from build123d import *

# Parameters (mm, degrees)
F1_DEPTH = 38.1
F3_DEPTH = 6.35


# Not quite as in the source:
# - the program builds the solid bodies; features that only make, move or delete a surface that nothing else refers to are left out


with BuildPart() as f1:
    # F0 (on Right) → F1 (new body)
    with BuildSketch(Plane.YZ):
        Polygon((12.7, 0), (25.4, 0), (25.4, 25.4), (12.7, 12.7), align=None)
    extrude(amount=F1_DEPTH)

    # F2 (on Right) → F3 (join)
    with BuildSketch(Plane.YZ):
        Polygon((12.7, 12.7), (0, 0), (12.7, 0), align=None)
    extrude(amount=F3_DEPTH)


solid = f1.part
Build history of the part. All positions in model axes, mm. A direction names the side the tool comes from. Coordinates: 2 decimals unless noted, no trailing zeros. Write each loop counter-clockwise with the first axis right and the second up, starting at its lowest first coordinate (ties: lowest second). Pieces come first, ordered by that corner, then holes.
(1) Mould opens along Y. For faces 3 (the flat face through (15, 18, 0)), 4 (the flat face through (19, 25.4, 13)), 5 (the flat face through (15, 16, 16)) say: pulls with the +Y half, pulls with the -Y half, needs draft (parallel to the pull), parting line crosses it, or undercut.
(2) Pin check, flat tips, straight feed: pin 1 Ø12 at (x, y) = (22.5, 13) entering from +Z; pin 2 Ø6 at (x, y) = (28, 17.5) entering from +Z; pin 3 Ø4 at (x, z) = (20.5, 14.5) entering from -Y; pin 4 Ø5 at (x, y) = (29.5, 14) entering from -Z. Stop position of each tip, or through.
(3) Drill centre lines: line 1 (Y direction, x = 36, z = 1.75); line 2 (X direction, y = 4.25, z = 3); line 3 (Y direction, x = 2, z = 10.5). Where is each one in solid material? Low to high.
(4) 3-axis set-ups, long thin cutter, end or side, ignore diameter. For faces 1 (the flat face through (6.35, 9, 4)), 2 (the flat face through (0, 18, 7)): which of +Z, -Z, +X, -X, +Y, -Y reach the whole face in a straight line?
(5) Cut at A-A on z = 12.25. List the corners of the cut face in (x, y).
(6) Cut at B-B on y = 20.5. List the corners of the cut face in (x, z).
(7) Cut at C-C on x = 14. List the corners of the cut face in (y, z).
(8) Cut at D-D on z = 8. List the corners of the cut face in (x, y), and give its area (3 significant figures).
Working result:
1. face 3: needs draft
1. face 4: pulls with the +Y half
1. face 5: pulls with the -Y half
2. pin 1: stops at z = 19
2. pin 2: stops at z = 20.5
2. pin 3: stops at y = 12.7
2. pin 4: stops at z = 0
3. line 1: y = 12.7 to 25.4
3. line 2: x = 0 to 6.35
3. line 3: y = 10.5 to 25.4
4. face 1: +Z, -Z, +X, -Y
4. face 2: +Z, -Z, -X, +Y, -Y
5. outline: (0, 12.25) - (6.35, 12.25) - (6.35, 12.7) - (38.1, 12.7) - (38.1, 25.4) - (0, 25.4) - close
6. outline: (0, 0) - (38.1, 0) - (38.1, 20.5) - (0, 20.5) - close
7. outline: (12.7, 0) - (25.4, 0) - (25.4, 25.4) - (12.7, 12.7) - close
8. outline: (0, 8) - (6.35, 8) - (6.35, 12.7) - (38.1, 12.7) - (38.1, 25.4) - (0, 25.4) - close
8. area: 514 mm2
